Autodesk Inventor part; units mm, degrees
ref_plane "YZ Plane" through (0, 0, 0) normal (1, 0, 0) x (0, 1, 0)
ref_plane "XZ Plane" through (0, 0, 0) normal (0, 1, 0) x (-1, 0, 0)
ref_plane "XY Plane" through (0, 0, 0) normal (0, 0, 1) x (1, 0, 0)
sketch "Sketch1" plane through (0, 0, 0) normal (0, 0, 1) x (1, 0, 0)
  circle A0 centre (0, 0) radius 20
  line L0 (-33.2, 28.2) -> (33.2, 28.2)
  line L1 (33.2, 28.2) -> (33.2, -33.2)
  line L2 (33.2, -33.2) -> (-33.2, -33.2)
  line L3 (-33.2, -33.2) -> (-33.2, 28.2)
  circle A1 centre (-23.7, 23.7) radius 2.5
  circle A2 centre (23.7, 23.7) radius 2.5
  circle A3 centre (23.7, -23.7) radius 2.5
  circle A4 centre (-23.7, -23.7) radius 2.5
  line L4 (-33.2, 28.2) -> (-33.2, 91.3)
  line L5 (-33.2, 91.3) -> (33.2, 91.3)
  line L6 (33.2, 91.3) -> (33.2, 28.2)
  circle A5 centre (-13.2, 78.8) radius 4
  circle A6 centre (13.2, 78.8) radius 4
  dimension "d0" = 40
  dimension "d1" = 66.4
  dimension "d2" = 61.4
  dimension "d3" = 33.2
  dimension "d4" = 28.2
  dimension "d5" = 5
  dimension "d6" = 5
  dimension "d7" = 5
  dimension "d8" = 5
  dimension "d9" = 47.4
  dimension "d10" = 47.4
  dimension "d11" = 47.4
  dimension "d12" = 47.4
  dimension "d13" = 4.5
  dimension "d14" = 9.5
  dimension "d15" = 9.5
  dimension "d16" = 9.5
  dimension "d19" = 63.1
  dimension "d20" = 8
  dimension "d21" = 8
  dimension "d23" = 20
  dimension "d24" = 20
  dimension "d27" = 12.5
  dimension "d28" = 12.5
extrude "Extrusion1" add sketch "Sketch1" along normal blind 12
properties part number "NEMA 23 Holder"
Here's how the part is built. I have some questions about the finished solid (model axes, mm). Give positions to 0.01 mm unless a question says otherwise; leave off trailing zeros. Write each loop counter-clockwise with the first axis right and the second up, starting at its lowest first coordinate (ties: lowest second). Pieces come first, ordered by that corner, then holes. Notation, with made-up numbers: (74.25, -19) -> (100.25, -19) arc R22 cw to (100.25, 6) -> close; hole circle Ø3 at (6, -15). An arc over 180 degrees is marked (long way). Use one line per item in the form item = value. Start each with the question number.
1. If I drill on L1, parallel to Y at x = -23.7, z = 7.25; L2, parallel to Y at x = 16.5, z = 7.75; L3, parallel to Y at x = 0, z = 3.75, over which ranges is the centre line in solid material (lowest first)?
2. Imagine slicing it at C-C on z = 2. List the corners of the cut face in (x, y) for me.
3. Will this pin go through, and if not, where does the flat tip stop? pin 1 Ø4.5 at (x, y) = (-23.7, -23.7) entering from +Z.
4. Imagine slicing it at A-A on y = 78.8. List the corners of the cut face in (x, z) for me, plus the area to 3 significant figures.
5. Imagine slicing it at D-D on x = -23.7. List the corners of the cut face in (y, z) for me.
6. Thinking about a two-plate mould opening in X: for faces 1 (the face through (-33.2, 28, 6)), 2 (the face through (0, 30, 12)), 3 (the face through (-22.55, 25.92, 5.92)), 4 (the face through (21.2, 23.6, 5.9)), which applies, +X half, -X half, draft (parallel to the pull), parting line (faces both ways), or undercut?
7. Imagine slicing it at B-B on x = 0. List the corners of the cut face in (y, z) for me.
Entries:
q1.L1 = -33.2 to -26.2, -21.2 to 21.2, 26.2 to 91.3
q1.L2 = -33.2 to -11.3, 11.3 to 76.54, 81.06 to 91.3
q1.L3 = -33.2 to -20, 20 to 91.3
q2.outline = (-33.2, -33.2) -> (33.2, -33.2) -> (33.2, 91.3) -> (-33.2, 91.3) -> close; hole circle Ø5 at (-23.7, -23.7); hole circle Ø5 at (-23.7, 23.7); hole circle Ø40 at (0, 0); hole circle Ø8 at (-13.2, 78.8); hole circle Ø8 at (13.2, 78.8); hole circle Ø5 at (23.7, -23.7); hole circle Ø5 at (23.7, 23.7)
q3.pin_1 = through
q4.outline = (-33.2, 0) -> (-17.2, 0) -> (-17.2, 12) -> (-33.2, 12) -> close; (-9.2, 0) -> (9.2, 0) -> (9.2, 12) -> (-9.2, 12) -> close; (17.2, 0) -> (33.2, 0) -> (33.2, 12) -> (17.2, 12) -> close
q4.area = 605 mm²
q5.outline = (-33.2, 0) -> (-26.2, 0) -> (-26.2, 12) -> (-33.2, 12) -> close; (-21.2, 0) -> (21.2, 0) -> (21.2, 12) -> (-21.2, 12) -> close; (26.2, 0) -> (91.3, 0) -> (91.3, 12) -> (26.2, 12) -> close
q6.face_1 = -X half
q6.face_2 = draft
q6.face_3 = undercut
q6.face_4 = undercut
q7.outline = (-33.2, 0) -> (-20, 0) -> (-20, 12) -> (-33.2, 12) -> close; (20, 0) -> (91.3, 0) -> (91.3, 12) -> (20, 12) -> close
